Geometry check sheet. Reference: the model listing, model coordinates, mm. A direction names the side the tool comes from. Give positions to 0.01 mm unless a question says otherwise; leave off trailing zeros. Write each loop counter-clockwise with the first axis right and the second up, starting at its lowest first coordinate (ties: lowest second). Pieces come first, ordered by that corner, then holes. Notation, with made-up numbers: M -32,28.25 L -7,28.25 A7 ccw -7,35.25 Z; hole C -1.75,3 d11. An arc over 180 degrees is marked long. Use one line per item in the form item = value. Start each with the question number.
```python
from build123d import *

# Parameters (mm, degrees)
SKETCH1_W                               = 77
SKETCH1_H                               = 60
BOSS_EXTRUDE1_DEPTH                     = 8
SKETCH3_W                               = 60
SKETCH3_H                               = 26
BOSS_EXTRUDE2_DEPTH                     = 9
SKETCH4_R                               = 4
CUT_EXTRUDE2_DEPTH                      = 107.395488626
SKETCH5_W                               = 31
SKETCH5_H                               = 14
BOSS_EXTRUDE3_DEPTH                     = 30
CUT_EXTRUDE3_DEPTH                      = 108.930533215
FILLET1_R                               = 10
SKETCH8_R                               = 1.75
F_3_5MM_SCREW_HOLE_FOR_TENSIONING_DEPTH = 93.012227514


with BuildPart() as part:
    # Sketch1 → Boss-Extrude1 (new body)
    with BuildSketch(Plane(origin=(0, 0, 0), x_dir=(1, 0, 0), z_dir=(0, 1, 0))):
        with Locations((38.5, 30)):
            Rectangle(SKETCH1_W, SKETCH1_H)
    extrude(amount=BOSS_EXTRUDE1_DEPTH)

    # Sketch3 → Boss-Extrude2 (add)
    with BuildSketch(Plane(origin=(77, 0, 0), x_dir=(0, 0, -1), z_dir=(1, 0, 0))):
        with Locations((30, -5)):
            Rectangle(SKETCH3_W, SKETCH3_H)
    extrude(amount=BOSS_EXTRUDE2_DEPTH)

    # Sketch4 → Cut-Extrude2 (cut, through all)
    with BuildSketch(Plane(origin=(86, 0, 0), x_dir=(0, 0, -1), z_dir=(1, 0, 0))):
        with Locations((8.5, -7)):
            Circle(SKETCH4_R)
        with Locations(Location((51.5, -7, 0), (0, 0, 180))):
            Circle(SKETCH4_R)
    extrude(amount=-CUT_EXTRUDE2_DEPTH, mode=Mode.SUBTRACT)

    # Sketch5 → Boss-Extrude3 (add)
    with BuildSketch(Plane(origin=(0, 8, 0), x_dir=(1, 0, 0), z_dir=(0, 1, 0))):
        with Locations((43, 46)):
            Rectangle(SKETCH5_W, SKETCH5_H)
    extrude(amount=BOSS_EXTRUDE3_DEPTH)

    # Sketch6 → Cut-Extrude3 (cut, through all)
    with BuildSketch(Plane(origin=(0, 0, -53), x_dir=(-1, 0, 0), z_dir=(0, 0, -1))):
        with BuildLine():
            Line((-49.500000097, 30.65), (-36.499999903, 30.65))
            ThreePointArc((-36.499999903, 30.65), (-33.999999903, 28.15), (-36.499999903, 25.65))
            Line((-36.499999903, 25.65), (-49.500000097, 25.65))
            ThreePointArc((-49.500000097, 25.65), (-52.000000097, 28.15), (-49.500000097, 30.65))
        make_face()
    extrude(amount=-CUT_EXTRUDE3_DEPTH, mode=Mode.SUBTRACT)

    # Fillet1
    # the kernel refuses this fillet: 10 mm, written as the material it adds along each edge
    with BuildSketch(Plane(origin=(58.5, 8, -53), x_dir=(0, 0, -1), z_dir=(-1, 0, 0))) as fillet1_piece_1:
        with BuildLine():
            CenterArc((10, -9.539392014), FILLET1_R, 107.457603124, 72.542396876)
            Line((0, -9.539392014), (-0.2, -9.539392014))
            Line((-0.2, -9.539392014), (-0.2, 0))
            Line((-0.2, 0), (0, 0.2))
            ThreePointArc((0, 0.2), (3.5, 0.2), (6.94, 0.19078784))
            Line((6.94, 0.19078784), (7, 0))
        make_face()
    extrude(amount=31)
    with BuildSketch(Plane(origin=(27.5, 8, -53), x_dir=(-1, 0, 0), z_dir=(0, 0, 1)), Plane(origin=(58.5, 8, -39), x_dir=(1, 0, 0), z_dir=(0, 0, -1))) as fillet1_piece_2:
        with BuildLine():
            CenterArc((FILLET1_R, -FILLET1_R), FILLET1_R, 90, 90)
            Line((0, -FILLET1_R), (-FILLET1_R * 0.02, -FILLET1_R))
            Line((-FILLET1_R * 0.02, -FILLET1_R), (-FILLET1_R * 0.02, FILLET1_R * 0.02))
            Line((-FILLET1_R * 0.02, FILLET1_R * 0.02), (FILLET1_R, FILLET1_R * 0.02))
            Line((FILLET1_R, FILLET1_R * 0.02), (FILLET1_R, 0))
        make_face()
    extrude(amount=14)
    with BuildSketch(Plane(origin=(27.5, 8, -39), x_dir=(0, 0, 1), z_dir=(1, 0, 0))) as fillet1_piece_3:
        with BuildLine():
            CenterArc((FILLET1_R, -FILLET1_R), FILLET1_R, 90, 90)
            Line((0, -FILLET1_R), (-FILLET1_R * 0.02, -FILLET1_R))
            Line((-FILLET1_R * 0.02, -FILLET1_R), (-FILLET1_R * 0.02, FILLET1_R * 0.02))
            Line((-FILLET1_R * 0.02, FILLET1_R * 0.02), (FILLET1_R, FILLET1_R * 0.02))
            Line((FILLET1_R, FILLET1_R * 0.02), (FILLET1_R, 0))
        make_face()
    extrude(amount=31)
    with BuildSketch(Plane(origin=(82.348480035, 8, -53), x_dir=(0, 0, -1), z_dir=(-1, 0, 0))) as fillet1_piece_4a_section:
        with BuildLine():
            CenterArc((10, -9.539392014), FILLET1_R, 107.457603124, 72.542396876)
            Line((0, -9.539392014), (-0.2, -9.539392014))
            Line((-0.2, -9.539392014), (-0.2, 0))
            Line((-0.2, 0), (0, 0.2))
            ThreePointArc((0, 0.2), (3.5, 0.2), (6.94, 0.19078784))
            Line((6.94, 0.19078784), (7, 0))
        make_face()
    fillet1_piece_4a = extrude(amount=54.848480035, mode=Mode.PRIVATE)
    fillet1_piece_4a = split(fillet1_piece_4a, bisect_by=Plane(origin=(58.5, 10.271225878, -54.787817996), z_dir=(1, 0, 0)), keep=Keep.TOP, mode=Mode.PRIVATE)
    with BuildSketch(Plane(origin=(58.5, 8, -39), x_dir=(1, 0, 0), z_dir=(0, 0, -1))) as fillet1_piece_4b_section:
        with BuildLine():
            CenterArc((FILLET1_R, -FILLET1_R), FILLET1_R, 90, 90)
            Line((0, -FILLET1_R), (-FILLET1_R * 0.02, -FILLET1_R))
            Line((-FILLET1_R * 0.02, -FILLET1_R), (-FILLET1_R * 0.02, FILLET1_R * 0.02))
            Line((-FILLET1_R * 0.02, FILLET1_R * 0.02), (FILLET1_R, FILLET1_R * 0.02))
            Line((FILLET1_R, FILLET1_R * 0.02), (FILLET1_R, 0))
        make_face()
    fillet1_piece_4b = extrude(amount=39, mode=Mode.PRIVATE)
    fillet1_piece_4b = split(fillet1_piece_4b, bisect_by=Plane(origin=(60.763951143, 10.263951143, -60), z_dir=(0, 0, 1)), keep=Keep.TOP, mode=Mode.PRIVATE)
    fillet1_piece_4b = split(fillet1_piece_4b, bisect_by=Plane(origin=(60.763951143, 10.263951143, -53), z_dir=(0, 0, -1)), keep=Keep.TOP, mode=Mode.PRIVATE)
    fillet1_piece_4 = fillet1_piece_4a & fillet1_piece_4b
    add(fillet1_piece_4)
    with BuildSketch(Plane(origin=(58.5, 8, -53), x_dir=(0, 0, -1), z_dir=(-1, 0, 0))) as fillet1_piece_5a_section:
        with BuildLine():
            CenterArc((10, -9.539392014), FILLET1_R, 107.457603124, 72.542396876)
            Line((0, -9.539392014), (-0.2, -9.539392014))
            Line((-0.2, -9.539392014), (-0.2, 0))
            Line((-0.2, 0), (0, 0.2))
            ThreePointArc((0, 0.2), (3.5, 0.2), (6.94, 0.19078784))
            Line((6.94, 0.19078784), (7, 0))
        make_face()
    fillet1_piece_5a = extrude(amount=54.848480035, mode=Mode.PRIVATE)
    fillet1_piece_5a = split(fillet1_piece_5a, bisect_by=Plane(origin=(27.5, 10.271225878, -54.787817996), z_dir=(-1, 0, 0)), keep=Keep.TOP, mode=Mode.PRIVATE)
    with BuildSketch(Plane(origin=(27.5, 8, -78), x_dir=(-1, 0, 0), z_dir=(0, 0, 1))) as fillet1_piece_5b_section:
        with BuildLine():
            CenterArc((FILLET1_R, -FILLET1_R), FILLET1_R, 90, 90)
            Line((0, -FILLET1_R), (-FILLET1_R * 0.02, -FILLET1_R))
            Line((-FILLET1_R * 0.02, -FILLET1_R), (-FILLET1_R * 0.02, FILLET1_R * 0.02))
            Line((-FILLET1_R * 0.02, FILLET1_R * 0.02), (FILLET1_R, FILLET1_R * 0.02))
            Line((FILLET1_R, FILLET1_R * 0.02), (FILLET1_R, 0))
        make_face()
    fillet1_piece_5b = extrude(amount=39, mode=Mode.PRIVATE)
    fillet1_piece_5b = split(fillet1_piece_5b, bisect_by=Plane(origin=(25.236048857, 10.263951143, -60), z_dir=(0, 0, 1)), keep=Keep.TOP, mode=Mode.PRIVATE)
    fillet1_piece_5b = split(fillet1_piece_5b, bisect_by=Plane(origin=(25.236048857, 10.263951143, -53), z_dir=(0, 0, -1)), keep=Keep.TOP, mode=Mode.PRIVATE)
    fillet1_piece_5 = fillet1_piece_5a & fillet1_piece_5b
    add(fillet1_piece_5)
    with BuildSketch(Plane(origin=(27.5, 8, -53), x_dir=(-1, 0, 0), z_dir=(0, 0, 1))) as fillet1_piece_6a_section:
        with BuildLine():
            CenterArc((FILLET1_R, -FILLET1_R), FILLET1_R, 90, 90)
            Line((0, -FILLET1_R), (-FILLET1_R * 0.02, -FILLET1_R))
            Line((-FILLET1_R * 0.02, -FILLET1_R), (-FILLET1_R * 0.02, FILLET1_R * 0.02))
            Line((-FILLET1_R * 0.02, FILLET1_R * 0.02), (FILLET1_R, FILLET1_R * 0.02))
            Line((FILLET1_R, FILLET1_R * 0.02), (FILLET1_R, 0))
        make_face()
    fillet1_piece_6a = extrude(amount=39, mode=Mode.PRIVATE)
    fillet1_piece_6a = split(fillet1_piece_6a, bisect_by=Plane(origin=(25.236048857, 10.263951143, -39), z_dir=(0, 0, 1)), keep=Keep.TOP, mode=Mode.PRIVATE)
    with BuildSketch(Plane(origin=(2.5, 8, -39), x_dir=(0, 0, 1), z_dir=(1, 0, 0))) as fillet1_piece_6b_section:
        with BuildLine():
            CenterArc((FILLET1_R, -FILLET1_R), FILLET1_R, 90, 90)
            Line((0, -FILLET1_R), (-FILLET1_R * 0.02, -FILLET1_R))
            Line((-FILLET1_R * 0.02, -FILLET1_R), (-FILLET1_R * 0.02, FILLET1_R * 0.02))
            Line((-FILLET1_R * 0.02, FILLET1_R * 0.02), (FILLET1_R, FILLET1_R * 0.02))
            Line((FILLET1_R, FILLET1_R * 0.02), (FILLET1_R, 0))
        make_face()
    fillet1_piece_6b = extrude(amount=56, mode=Mode.PRIVATE)
    fillet1_piece_6b = split(fillet1_piece_6b, bisect_by=Plane(origin=(27.5, 10.263951143, -36.736048857), z_dir=(-1, 0, 0)), keep=Keep.TOP, mode=Mode.PRIVATE)
    fillet1_piece_6 = fillet1_piece_6a & fillet1_piece_6b
    add(fillet1_piece_6)
    with BuildSketch(Plane(origin=(27.5, 8, -39), x_dir=(0, 0, 1), z_dir=(1, 0, 0))) as fillet1_piece_7a_section:
        with BuildLine():
            CenterArc((FILLET1_R, -FILLET1_R), FILLET1_R, 90, 90)
            Line((0, -FILLET1_R), (-FILLET1_R * 0.02, -FILLET1_R))
            Line((-FILLET1_R * 0.02, -FILLET1_R), (-FILLET1_R * 0.02, FILLET1_R * 0.02))
            Line((-FILLET1_R * 0.02, FILLET1_R * 0.02), (FILLET1_R, FILLET1_R * 0.02))
            Line((FILLET1_R, FILLET1_R * 0.02), (FILLET1_R, 0))
        make_face()
    fillet1_piece_7a = extrude(amount=56, mode=Mode.PRIVATE)
    fillet1_piece_7a = split(fillet1_piece_7a, bisect_by=Plane(origin=(58.5, 10.263951143, -36.736048857), z_dir=(1, 0, 0)), keep=Keep.TOP, mode=Mode.PRIVATE)
    with BuildSketch(Plane(origin=(58.5, 8, -14), x_dir=(1, 0, 0), z_dir=(0, 0, -1))) as fillet1_piece_7b_section:
        with BuildLine():
            CenterArc((FILLET1_R, -FILLET1_R), FILLET1_R, 90, 90)
            Line((0, -FILLET1_R), (-FILLET1_R * 0.02, -FILLET1_R))
            Line((-FILLET1_R * 0.02, -FILLET1_R), (-FILLET1_R * 0.02, FILLET1_R * 0.02))
            Line((-FILLET1_R * 0.02, FILLET1_R * 0.02), (FILLET1_R, FILLET1_R * 0.02))
            Line((FILLET1_R, FILLET1_R * 0.02), (FILLET1_R, 0))
        make_face()
    fillet1_piece_7b = extrude(amount=39, mode=Mode.PRIVATE)
    fillet1_piece_7b = split(fillet1_piece_7b, bisect_by=Plane(origin=(60.763951143, 10.263951143, -39), z_dir=(0, 0, 1)), keep=Keep.TOP, mode=Mode.PRIVATE)
    fillet1_piece_7 = fillet1_piece_7a & fillet1_piece_7b
    add(fillet1_piece_7)

    # Sketch8 → 3.5mm screw hole for tensioning (cut, through all)
    with BuildSketch(Plane(origin=(58.5, 0, 0), x_dir=(0, 0, -1), z_dir=(1, 0, 0))):
        with Locations((46, 28.15)):
            Circle(SKETCH8_R)
    extrude(amount=-F_3_5MM_SCREW_HOLE_FOR_TENSIONING_DEPTH, mode=Mode.SUBTRACT)


solid = part.part
```
(1) Tool access check on faces 1 (the flat face through (43, 25.65, -46)), 2 (the flat face through (58.5, 30.1, -46.1)), 3 (the flat face through (77, -9, -30)), 4 (the flat face through (42, 8, -23)). Record the directions out of +Z, -Z, +X, -X, +Y, -Y that give a thin tool (end or side, any length) a straight path to the whole face; none if there is none.
(2) Depth check by flat-ended pin: pin 1 (4 mm diameter, centred on y = 30, z = -44, fed in from -X); pin 2 (22 mm diameter, centred on x = 50, y = 29, fed in from +Z); pin 3 (5 mm diameter, centred on y = -7, z = -51.5, fed in from +X); pin 4 (3 mm diameter, centred on x = 62.5, y = 7.5, fed in from +Z). Enter the tip coordinate at first touch or a pass-through.
(3) Sectioned sample at D-D, the plane z = -8.5. Record the boundary of the cut face in (x, y).
(4) Sectioned sample at B-B, the plane y = -7. Record the boundary of the cut face in (x, z).
(5) Thickness scan on probe 1 along Y at (x, z) = (38.5, -48.5); probe 2 along Y at (x, z) = (56.25, -46); probe 3 along Z at (x, y) = (30.25, 28.15). Record the ranges inside material, lowest first. Write a range as [from, to].
(6) Sectioned sample at C-C, the plane x = 30. Record the boundary of the cut face in (y, z).
(7) Sectioned sample at A-A, the plane z = -51.5. Record the boundary of the cut face in (x, y), plus the area to 3 significant figures.
(8) Draft check along Z on faces 5 (the flat face through (52, 1, -60)), 6 (the cylindrical face through (31.158, 27.48, -47.617)), 7 (the flat face through (52, 1, 0)). Enter one of: released by +Z, released by -Z, zero draft, split by the parting line, or undercut.
Numbers:
q1.face_1 = +Z, -Z
q1.face_2 = +Z, -Z, +X, +Y
q1.face_3 = +Z, -Z, -X, -Y
q1.face_4 = +Z, +Y
q2.pin_1 = 27.5
q2.pin_2 = -39
q2.pin_3 = through
q2.pin_4 = 0
q3.outline = M 0,0 L 77,0 L 77,-3 L 86,-3 L 86,8 L 0,8 Z; M 77,-18 L 86,-18 L 86,-11 L 77,-11 Z
q4.outline = M 77,-60 L 86,-60 L 86,-55.5 L 77,-55.5 Z; M 77,-47.5 L 86,-47.5 L 86,-12.5 L 77,-12.5 Z; M 77,-4.5 L 86,-4.5 L 86,0 L 77,0 Z
q5.probe_1 = [0, 25.65], [30.65, 38]
q5.probe_2 = [0, 26.4], [29.9, 38]
q5.probe_3 = [-53, -47.75], [-44.25, -39]
q6.outline = M 0,-60 L 8,-60 A10 cw 17.54,-53 L 38,-53 L 38,-39 L 18,-39 A10 cw 8,-29 L 8,0 L 0,0 Z; hole C 28.15,-46 d3.5
q7.outline = M 0,0 L 77,0 L 77,-3 L 86,-3 L 86,8 L 68.5,8 A10 cw 58.5,18 L 58.5,38 L 27.5,38 L 27.5,18 A10 cw 17.5,8 L 0,8 Z; M 77,-18 L 86,-18 L 86,-11 L 77,-11 Z; hole M 36.5,25.65 L 49.5,25.65 A2.5 ccw 49.5,30.65 L 36.5,30.65 A2.5 ccw Z
q7.area = 1,670 mm2
q8.face_5 = released by -Z
q8.face_6 = undercut
q8.face_7 = released by +Z
